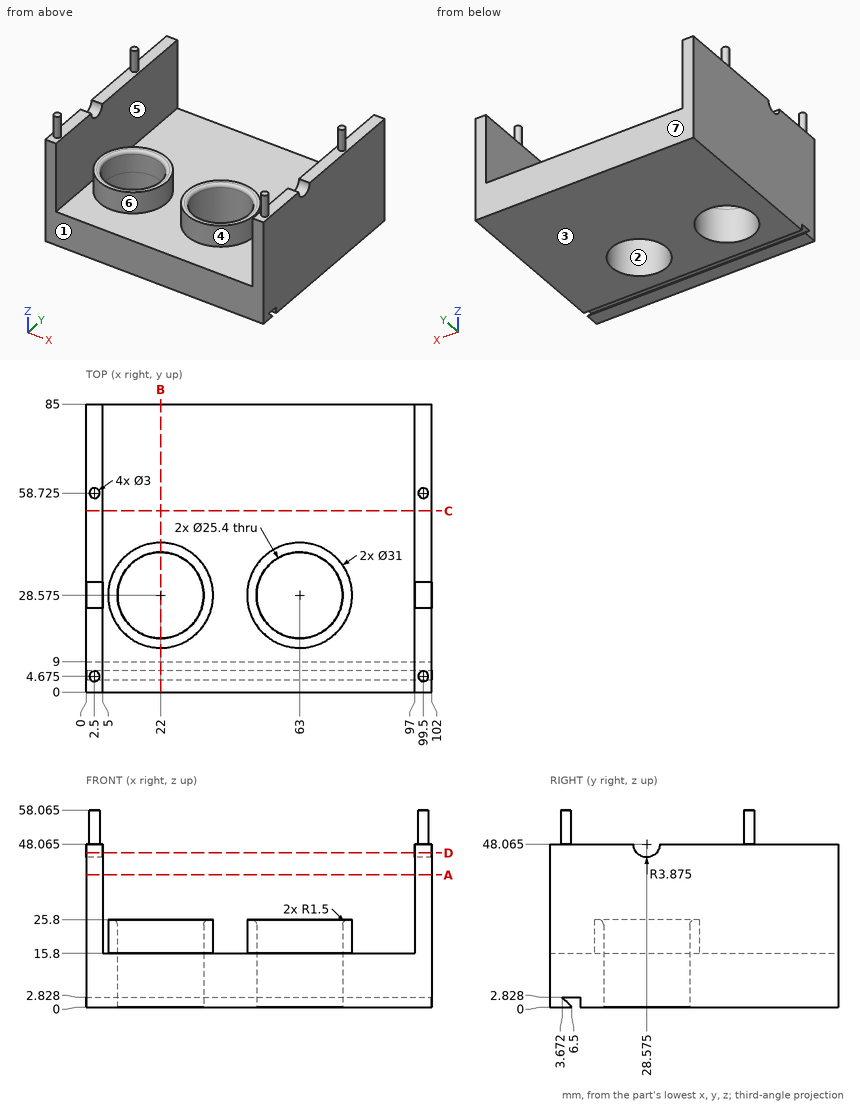
Part print with two shaded views. Sizes in mm from the minimum x, y, z corner. A direction names the side the tool comes from. Give positions to 0.01 mm unless a question says otherwise; leave off trailing zeros. Order: outer loops, then holes, each group sorted by start corner. A loop starts at its lowest first (then second) coordinate and runs counter-clockwise, first axis right, second up.
1) Mould opens along Y. For the marked faces 1, 2, 3 and 4 say: +Y half, -Y half, draft (parallel to the pull), parting line (faces both ways), or undercut.
2) 3-axis set-ups, long thin cutter, end or side, ignore diameter. For the marked faces 5, 6 and 7: which of +Z, -Z, +X, -X, +Y, -Y reach the whole face in a straight line?
3) Saw through at B-B, the plane x = 22. Write the cut outline in (y, z) (1 decimal).
4) Saw through at D-D, the plane z = 45.5. Write the cut outline in (x, y).
5) Wall check: probe 1 along Y at (x, z) = (22, 5) (1 decimal); probe 2 along Y at (x, z) = (22, 20) (1 decimal); probe 3 along X at (y, z) = (78, 18.5). Give the ranges that are in metal, low to high.
6) Saw through at C-C, the plane y = 53.5. Write the cut outline in (x, z) (1 decimal).
7) Saw through at A-A, the plane z = 39. Write the cut outline in (x, y), then the cut area to 3 significant figures.
8) Pin check, flat tips, straight feed: pin 1 (9.5 mm diameter, centred on x = 15, y = 22, fed in from +Z); pin 2 (5.5 mm diameter, centred on x = 99, y = 65, fed in from +Z) (3 decimals); pin 3 (20.5 mm diameter, centred on x = 63, y = 28.575, fed in from -Z); pin 4 (8 mm diameter, centred on x = 71, z = 20, fed in from -Y). Stop position of each tip, or through.
Computed:
1. face 1: -Y half
1. face 2: undercut
1. face 3: draft
1. face 4: parting line
2. face 5: +Z, +Y, -Y
2. face 6: +Z
2. face 7: +Z, -Z, +X, -X, +Y
3. outline: (0, 0) - (6.5, 0) - (3.7, 2.8) - (9, 2.8) - (9, 0) - (15.9, 0) - (15.9, 24.3) arc R1.5 ccw to (14.4, 25.8) - (13.1, 25.8) - (13.1, 15.8) - (0, 15.8) - close; (41.3, 0) - (85, 0) - (85, 15.8) - (44.1, 15.8) - (44.1, 25.8) - (42.8, 25.8) arc R1.5 ccw to (41.3, 24.3) - close
4. outline: (0, 0) - (5, 0) - (5, 25.67) - (0, 25.67) - close; (0, 31.48) - (5, 31.48) - (5, 85) - (0, 85) - close; (97, 0) - (102, 0) - (102, 25.67) - (97, 25.67) - close; (97, 31.48) - (102, 31.48) - (102, 85) - (97, 85) - close
5. probe 1: y = 0 to 15.9, 41.3 to 85
5. probe 2: y = 13.1 to 15.9, 41.3 to 44.1
5. probe 3: x = 0 to 5, 97 to 102
6. outline: (0, 0) - (102, 0) - (102, 48.1) - (97, 48.1) - (97, 15.8) - (5, 15.8) - (5, 48.1) - (0, 48.1) - close
7. outline: (0, 0) - (5, 0) - (5, 85) - (0, 85) - close; (97, 0) - (102, 0) - (102, 85) - (97, 85) - close
7. area: 850 mm2
8. pin 1: stops at z = 25.8
8. pin 2: stops at z = 48.065
8. pin 3: passes through
8. pin 4: stops at y = 13.6
